Input: part model. Units: mm. Frame: model coordinates. Face numbers are marked on the shaded views. Give positions to 0.01 mm unless a question says otherwise; leave off trailing zeros. Loops run counter-clockwise (first coordinate to the right, second up) from the corner with the lowest first, then second, coordinate; pieces in that order, holes last. Notation, with made-up numbers: M -26.5,89 L 24.5,89 A16 cw 24.5,95 Z; hole C 67.5,17 d6. An arc over 180 degrees is marked long. Use CSV: the item, a comma, the result in double quotes. Start each with the question number.
Q1. Pull-direction query (Y, two-part tool) for the marked faces 1, 2 and 3; classes: released by +Y, released by -Y, zero draft, split by the parting line, or undercut.
Q2. Section B-B, the plane y = 8.25. Output: boundary loops of the cut face in (x, z) (3 decimals), plus the area to 3 significant figures.
Q3. Section C-C, the plane z = 16. Output: boundary loops of the cut face in (x, y), plus the area to 3 significant figures.
Q4. Material intervals for line 1 along Z through (x, y) = (0, 14.45); line 2 along Y through (x, z) = (0.25, 19); line 3 along Z through (x, y) = (-1.5, 3.5), sorted ascending.
Q5. Section D-D, the plane x = 0. State how many separate pieces and enclosed holes the cut face has, plus the area to 3 significant figures.
Q6. Section A-A, the plane y = 13.75. Output: boundary loops of the cut face in (x, z), plus the area to 3 significant figures.
Q7. Pin query (flat end, axial travel): pin 1 (2 mm diameter, centred on x = -0.5, y = -1.5, fed in from -Z); pin 2 (2.5 mm diameter, centred on x = 0, z = 6.5, fed in from +Y); pin 3 (4 mm diameter, centred on x = 4.5, z = 16.5, fed in from -Y). Return the tip coordinate at first contact, or that it passes through.
from build123d import *

# Parameters (mm, degrees)
SKETCH1_R           = 3.15
BOSS_EXTRUDE1_DEPTH = 47.5
CUT_EXTRUDE1_DEPTH  = 4.2
FILLET1_R           = 1
CHAMFER1_SIZE       = 1
CHAMFER2_SIZE       = 1


with BuildPart() as part:
    # Sketch1 → Boss-Extrude1 (new body)
    with BuildSketch(Plane.XY):
        with BuildLine():
            Line((6.15, 0), (6.15, 16.75))
            Line((6.15, 16.75), (-6.15, 16.75))
            Line((-6.15, 16.75), (-6.15, 0))
            ThreePointArc((-6.15, 0), (0, -6.15), (6.15, 0))
        make_face()
        Circle(SKETCH1_R, mode=Mode.SUBTRACT)
    extrude(amount=BOSS_EXTRUDE1_DEPTH)

    # Sketch4 → Cut-Extrude1 (cut)
    with BuildSketch(Plane(origin=(0, 11.75, 0), x_dir=(1, 0, 0), z_dir=(0, 1, 0))):
        Polygon((-3.204293994, -41), (-1.602146997, -43.775), (1.602146997, -43.775), (6.15, -43.775), (6.15, -38.225), (1.602146997, -38.225), (-1.602146997, -38.225), align=None)
    cut_extrude1 = extrude(amount=-CUT_EXTRUDE1_DEPTH, mode=Mode.SUBTRACT)

    # Sketch7 → M3 Clearance Hole1 (revolve, cut)
    with BuildSketch(Plane(origin=(0, 16.75, 41), x_dir=(0, 0, 1), z_dir=(1, 0, 0))):
        Polygon((0, 0), (0, 17.770463052), (1.7, 16.749), (1.7, 0.025), (1.725, 0), align=None)
    m3_clearance_hole1 = revolve(axis=Axis((0, 23.1, 41), (0, -1, 0)), mode=Mode.SUBTRACT)

    # Mirror1: Cut-Extrude1, M3 Clearance Hole1 across plane
    add(cut_extrude1.mirror(Plane(origin=(0, 0, 23.75), x_dir=(1, 0, 0), z_dir=(0, 0, -1))), mode=Mode.SUBTRACT)
    add(m3_clearance_hole1.mirror(Plane(origin=(0, 0, 23.75), x_dir=(1, 0, 0), z_dir=(0, 0, -1))), mode=Mode.SUBTRACT)

    # Fillet1
    fillet1_edges = [part.edges().sort_by_distance(p)[0] for p in [
        (6.15, 9.65, 38.225),
        (6.15, 9.65, 43.775),
        (6.15, 9.65, 3.725),
        (6.15, 9.65, 9.275),
    ]]
    fillet(fillet1_edges, radius=FILLET1_R)

    # Chamfer1
    chamfer1_edges = [part.edges().sort_by_distance(p)[0] for p in [
        (-6.15, 8.375, 47.5),
        (0, -6.15, 47.5),
        (-6.15, 8.375, 0),
        (6.15, 8.375, 0),
        (0, -6.15, 0),
        (-6.15, 16.75, 23.75),
        (6.15, 16.75, 23.75),
        (6.15, 8.375, 47.5),
    ]]
    chamfer(chamfer1_edges, length=CHAMFER1_SIZE)

    # Chamfer2
    chamfer2_edges = [part.edges().sort_by_distance(p)[0] for p in [
        (-3.15, 0, 0),
        (-3.15, 0, 47.5),
    ]]
    chamfer(chamfer2_edges, length=CHAMFER2_SIZE)


solid = part.part
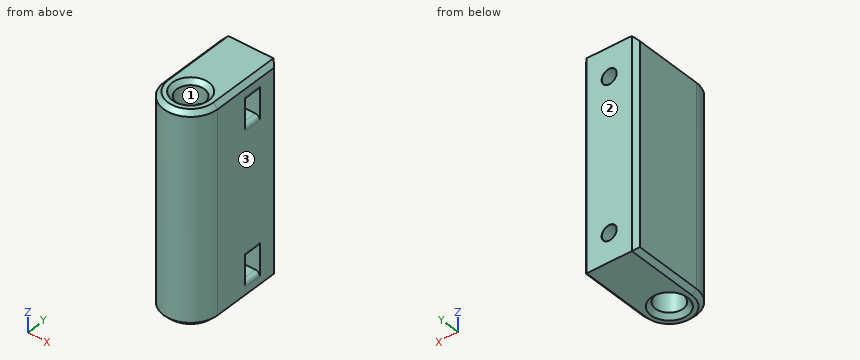
A:
1,face 1,"undercut"
1,face 2,"released by +Y"
1,face 3,"zero draft"
2,outline,"M -6.15,1 L -5.15,0 L 5.15,0 L 6.15,1 L 6.15,2.725 A1 ccw 5.15,3.725 L -1.602,3.725 L -3.204,6.5 L -1.602,9.275 L 5.15,9.275 A1 ccw 6.15,10.275 L 6.15,37.225 A1 ccw 5.15,38.225 L -1.602,38.225 L -3.204,41 L -1.602,43.775 L 5.15,43.775 A1 ccw 6.15,44.775 L 6.15,46.5 L 5.15,47.5 L -5.15,47.5 L -6.15,46.5 Z"
2,area,"486 mm^2"
3,outline,"M -6.15,0 A6.15 ccw 6.15,0 L 6.15,15.75 L 5.15,16.75 L -5.15,16.75 L -6.15,15.75 Z; hole C 0,0 d6.3"
3,area,"233 mm^2"
4,line 1,"0 to 4.8, 8.2 to 39.3, 42.7 to 47.5"
4,line 2,"-6.14 to -3.14, 3.14 to 16.75"
4,line 3,"0.34 to 5.7, 7.3 to 40.2, 41.8 to 47.16"
5,separate pieces,"4"
5,enclosed holes,"0"
5,area,"675 mm^2"
6,outline,"M -6.15,1 L -5.15,0 L 5.15,0 L 6.15,1 L 6.15,46.5 L 5.15,47.5 L -5.15,47.5 L -6.15,46.5 Z; hole C 0,6.5 d3.4; hole C 0,41 d3.4"
6,area,"564 mm^2"
7,pin 1,"through"
7,pin 2,"y = -2.89"
7,pin 3,"y = -5.62"
